Autodesk Inventor part; units mm, degrees
ref_plane "YZ Plane" through (0, 0, 0) normal (1, 0, 0) x (0, 1, 0)
ref_plane "XZ Plane" through (0, 0, 0) normal (0, 1, 0) x (-1, 0, 0)
ref_plane "XY Plane" through (0, 0, 0) normal (0, 0, 1) x (1, 0, 0)
sketch "Sketch1" plane through (0, 0, 0) normal (1, 0, 0) x (0, 1, 0)
  line L0 (0, 0) -> (0, 8.5)
  line L1 (0, 8.5) -> (3, 8.5)
  line L2 (3, 0) -> (4.3916, 2.4103)
  line L3 (3, 0) -> (5.7832, 0) construction
  line L4 (4.3916, 2.4103) -> (3, 4.8207)
  line L5 (3, 0) -> (0, 0)
  line L6 (3, 8.5) -> (3, 7.5231)
  line L7 (3, 7.5231) -> (3, 4.8207)
  dimension "d0" = 8.5
  dimension "d1" = 3
  dimension "d3" = 60
  dimension "d4" = 120
revolve "Revolution1" add sketch "Sketch1" angle 360 about axis through (0, 0, 0) along (0, 0, 1)
mirror "Mirror1" about plane through (0, 0, 0) normal (0, 0, -1)
shell "Shell1" thickness 1.5 removed faces 2 at (-1.0949, -0.5351, 8.5) at (-1.0949, -0.5351, -8.5)
properties part number "Flex_3DPrint"
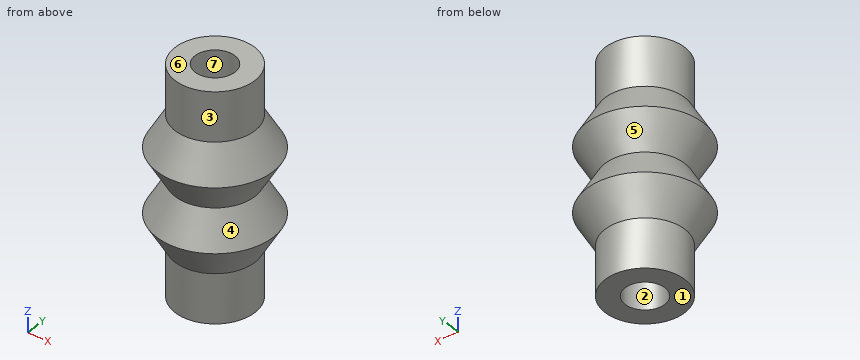
Input: part model. Units: mm. Frame: model coordinates. Face numbers are marked on the shaded views. A direction names the side the tool comes from. Give positions to 0.01 mm unless a question says otherwise; leave off trailing zeros. Order: outer loops, then holes, each group sorted by start corner. A loop starts at its lowest first (then second) coordinate and runs counter-clockwise, first axis right, second up. Notation, with made-up numbers: (70, -2.75) - (90, -2.75) arc R25 cw to (90, 15.25) - close; hole circle Ø7 at (88, 61). An arc over 180 degrees is marked (long way). Answer as a JSON object with one key per item and string values. Group by question number.
Q1. First-contact query: pin 1 Ø1.5 at (y, z) = (2.5, 0.5) entering from -X; pin 2 Ø5 at (y, z) = (-3, 5.5) entering from +X; pin 3 Ø5 at (y, z) = (1.5, 6) entering from +X. Flat tips, straight axial feed; report the tip coordinate or a pass-through.
Q2. Line query: probe 1 along X at (y, z) = (0, -6.8); probe 2 along Z at (x, y) = (1.75, 1.75). Output: solid intervals per line, ascending.
Q3. Cut plane C-C, the plane z = -6.25. Output: boundary loops of the cut face in (x, y).
Q4. Cut plane D-D, the plane x = -2. Count the separate pieces of the cut face and the enclosed holes in it, then the cut area to 3 significant figures.
Q5. Set-up query: the marked faces 1, 2, 3 and 4. Return all of +Z, -Z, +X, -X, +Y, -Y with unobstructed straight access to the full face (end or side cutting, diameter ignored); none if empty.
Q6. Cut plane A-A, the plane y = 0. Output: boundary loops of the cut face in (x, z), then the cut area to 3 significant figures.
Q7. Mould query, pull axis Y, two halves, no side actions, for the marked faces 5, 6 and 7. Classes: pulls with the +Y half, pulls with the -Y half, needs draft (parallel to the pull), parting line crosses it, or undercut.
Results:
{
 "1": {"pin 1": "x = -3.01", "pin 2": "x = 3.45", "pin 3": "x = 3.62"},
 "2": {"probe 1": "-3 to -1.5, 1.5 to 3", "probe 2": "-8.5 to -2.73, -2.09 to 2.09, 2.73 to 8.5"},
 "3": {"outline": "circle Ø6 at (0, 0); hole circle Ø3 at (0, 0)"},
 "4": {"separate pieces": "1", "enclosed holes": "2", "area": "82.2 mm^2"},
 "5": {"face 1": "-Z, +X, -X, +Y, -Y", "face 2": "-Z", "face 3": "+Z", "face 4": "none"},
 "6": {"outline": "(-4.39, -2.41) - (-3, -4.82) - (-3, -8.5) - (-1.5, -8.5) - (-1.5, -4.42) - (-2.66, -2.41) - (-1.27, 0) - (-2.66, 2.41) - (-1.5, 4.42) - (-1.5, 8.5) - (-3, 8.5) - (-3, 4.82) - (-4.39, 2.41) - (-3, 0) - close; (1.27, 0) - (2.66, -2.41) - (1.5, -4.42) - (1.5, -8.5) - (3, -8.5) - (3, -4.82) - (4.39, -2.41) - (3, 0) - (4.39, 2.41) - (3, 4.82) - (3, 8.5) - (1.5, 8.5) - (1.5, 4.42) - (2.66, 2.41) - close", "area": "55.3 mm^2"},
 "7": {"face 5": "parting line crosses it", "face 6": "needs draft", "face 7": "undercut"}
}
